For this review, take the finished solid that the model builds, in its own axes (mm). A direction names the side the tool comes from. Give positions to 0.01 mm unless a question says otherwise; leave off trailing zeros. One line per item, written item: value. Start each with the question number.
from build123d import *

# Parameters (mm, degrees)
SKETCH1_R            = 1
BOSS_EXTRUDE1_DEPTH  = 27.5
SKETCH2_R            = 1.01
BOSS_EXTRUDE2_DEPTH  = 13
SKETCH3_W            = 3.5
SKETCH3_H            = 13
BOSS_EXTRUDE3_DEPTH  = 49.6
SKETCH7_W            = 3.5
SKETCH7_H            = 49.5
BOSS_EXTRUDE6_DEPTH  = 5.5
SKETCH8_W            = 3.5
SKETCH8_H            = 49.5
BOSS_EXTRUDE7_DEPTH  = 14.5
FILLET2_R            = 4
BOSS_EXTRUDE8_DEPTH  = 29
BOSS_EXTRUDE9_DEPTH  = 0.2
BOSS_EXTRUDE11_DEPTH = 3.5
BOSS_EXTRUDE12_DEPTH = 1
FILLET2_OF_MIRROR1_R = 4
SKETCH15_R           = 1
CUT_EXTRUDE1_DEPTH   = 82.236014181
CHAMFER1_SIZE        = 0.5
FILLET3_R            = 0.5
FILLET4_R            = 0.5
FILLET6_R            = 0.7


with BuildPart() as part:
    # Sketch1 → Boss-Extrude1 (new body)
    with BuildSketch(Plane.XY):
        Circle(SKETCH1_R)
    boss_extrude1 = extrude(amount=BOSS_EXTRUDE1_DEPTH)


with BuildPart() as body_2:
    # Sketch2 → Boss-Extrude2 (new body)
    with BuildSketch(Plane.XY.offset(27.5)):
        with BuildLine():
            Line((-2.136524473, -0.092095918), (-4.5, -2.4))
            Line((-4.5, -2.4), (-1, -2.4))
            ThreePointArc((-1, -2.4), (-0.559963282, -2.050091796), (0, -2))
            ThreePointArc((0, -2), (1.487450997, 1.336970281), (-1.988677777, 0.212510468))
            ThreePointArc((-1.988677777, 0.212510468), (-2.036032236, 0.047311543), (-2.136524473, -0.092095918))
        make_face()
        Circle(SKETCH2_R, mode=Mode.SUBTRACT)
    boss_extrude2 = extrude(amount=-BOSS_EXTRUDE2_DEPTH)

    # Sketch3 → Boss-Extrude3 (add)
    with BuildSketch(Plane.XZ.offset(2.4)):
        with Locations((-2.75, 21)):
            Rectangle(SKETCH3_W, SKETCH3_H)
    boss_extrude3 = extrude(amount=BOSS_EXTRUDE3_DEPTH)

    # Sketch7 → Boss-Extrude6 (add)
    with BuildSketch(Plane.XY.offset(27.5)):
        with Locations((-2.75, -27.25)):
            Rectangle(SKETCH7_W, SKETCH7_H)
    boss_extrude6 = extrude(amount=BOSS_EXTRUDE6_DEPTH)

    # Sketch8 → Boss-Extrude7 (add)
    with BuildSketch(Plane(origin=(0, 0, 14.5), x_dir=(-1, 0, 0), z_dir=(0, 0, -1))):
        with Locations((2.75, -27.25)):
            Rectangle(SKETCH8_W, SKETCH8_H)
    boss_extrude7 = extrude(amount=BOSS_EXTRUDE7_DEPTH)

    # Fillet2
    fillet2_edges = [body_2.edges().sort_by_distance(p)[0] for p in [
        (-2.75, -2.5, 33),
        (-2.75, -52, 33),
    ]]
    fillet(fillet2_edges, radius=FILLET2_R)

    # Sketch10 → Boss-Extrude8 (add)
    with BuildSketch(Plane(origin=(0, 0, 0), x_dir=(-1, 0, 0), z_dir=(0, 0, -1))):
        Polygon((3.8, -52), (1, -52), (1, -54), (4.8, -54), (4.8, -53), (3.8, -53), align=None)
    boss_extrude8 = extrude(amount=-BOSS_EXTRUDE8_DEPTH)

    # Sketch11 → Boss-Extrude9 (add)
    with BuildSketch(Plane(origin=(-1, 0, 0), x_dir=(0, 0, -1), z_dir=(1, 0, 0))):
        with BuildLine():
            Line((0, -36.209762403), (-20, -36.209762403))
            ThreePointArc((-20, -36.209762403), (-21.414213562, -35.623975965), (-22, -34.209762403))
            Line((-22, -34.209762403), (-22, -25.209762403))
            ThreePointArc((-22, -25.209762403), (-21.414213562, -23.795548841), (-20, -23.209762403))
            Line((-20, -23.209762403), (0, -23.209762403))
            Line((0, -23.209762403), (0, -23.709762403))
            Line((0, -23.709762403), (-0.5, -23.709762403))
            Line((-0.5, -23.709762403), (-20, -23.709762403))
            ThreePointArc((-20, -23.709762403), (-21.060660172, -24.149102231), (-21.5, -25.209762403))
            Line((-21.5, -25.209762403), (-21.5, -34.209762403))
            ThreePointArc((-21.5, -34.209762403), (-21.060660172, -35.270422575), (-20, -35.709762403))
            Line((-20, -35.709762403), (-0.5, -35.709762403))
            Line((-0.5, -35.709762403), (0, -35.709762403))
            Line((0, -35.709762403), (0, -36.209762403))
        make_face()
    boss_extrude9 = extrude(amount=BOSS_EXTRUDE9_DEPTH)

    # Sketch13 → Boss-Extrude11 (add)
    with BuildSketch(Plane(origin=(-1, 0, 0), x_dir=(0, 0, -1), z_dir=(1, 0, 0))):
        with BuildLine():
            Line((-26.75, -5.5), (-0.75, -5.5))
            Line((-0.75, -5.5), (0, -5.5))
            Line((0, -5.5), (0, -4.75))
            Line((0, -4.75), (-26.75, -4.75))
            ThreePointArc((-26.75, -4.75), (-29.578427125, -5.921572875), (-30.75, -8.75))
            Line((-30.75, -8.75), (-30.75, -45.75))
            ThreePointArc((-30.75, -45.75), (-29.578427125, -48.578427125), (-26.75, -49.75))
            Line((-26.75, -49.75), (0, -49.75))
            Line((0, -49.75), (0, -49))
            Line((0, -49), (-0.75, -49))
            Line((-0.75, -49), (-26.75, -49))
            ThreePointArc((-26.75, -49), (-29.048097039, -48.048097039), (-30, -45.75))
            Line((-30, -45.75), (-30, -8.75))
            ThreePointArc((-30, -8.75), (-29.048097039, -6.451902961), (-26.75, -5.5))
        make_face()
    boss_extrude11 = extrude(amount=BOSS_EXTRUDE11_DEPTH)

    # Sketch14 → Boss-Extrude12 (add)
    with BuildSketch(Plane(origin=(2.5, 0, 0), x_dir=(0, 0, -1), z_dir=(1, 0, 0))):
        with BuildLine():
            Line((0, -49), (-26.75, -49))
            ThreePointArc((-26.75, -49), (-29.048097039, -48.048097039), (-30, -45.75))
            Line((-30, -45.75), (-30, -8.75))
            ThreePointArc((-30, -8.75), (-29.048097039, -6.451902961), (-26.75, -5.5))
            Line((-26.75, -5.5), (0, -5.5))
            Line((0, -5.5), (0, -4))
            Line((0, -4), (-26.75, -4))
            ThreePointArc((-26.75, -4), (-30.108757211, -5.391242789), (-31.5, -8.75))
            Line((-31.5, -8.75), (-31.5, -45.75))
            ThreePointArc((-31.5, -45.75), (-30.108757211, -49.108757211), (-26.75, -50.5))
            Line((-26.75, -50.5), (0, -50.5))
            Line((0, -50.5), (0, -49))
        make_face()
    boss_extrude12 = extrude(amount=BOSS_EXTRUDE12_DEPTH)


with BuildPart() as part_1:
    add(part.part)

    add(body_2.part)  # Mirror1 merges body 2
    # Mirror1: Boss-Extrude1, Boss-Extrude2, Boss-Extrude3, Boss-Extrude6, Boss-Extrude7, Boss-Extrude8, Boss-Extrude9, Boss-Extrude11, Boss-Extrude12 across plane
    add(boss_extrude1.mirror(Plane(origin=(0, 0, 0), x_dir=(1, 0, 0), z_dir=(0, 0, -1))))
    add(boss_extrude2.mirror(Plane(origin=(0, 0, 0), x_dir=(1, 0, 0), z_dir=(0, 0, -1))))
    add(boss_extrude3.mirror(Plane(origin=(0, 0, 0), x_dir=(1, 0, 0), z_dir=(0, 0, -1))))
    add(boss_extrude6.mirror(Plane(origin=(0, 0, 0), x_dir=(1, 0, 0), z_dir=(0, 0, -1))))
    add(boss_extrude7.mirror(Plane(origin=(0, 0, 0), x_dir=(1, 0, 0), z_dir=(0, 0, -1))))
    add(boss_extrude8.mirror(Plane(origin=(0, 0, 0), x_dir=(1, 0, 0), z_dir=(0, 0, -1))))
    add(boss_extrude9.mirror(Plane(origin=(0, 0, 0), x_dir=(1, 0, 0), z_dir=(0, 0, -1))))
    add(boss_extrude11.mirror(Plane(origin=(0, 0, 0), x_dir=(1, 0, 0), z_dir=(0, 0, -1))))
    add(boss_extrude12.mirror(Plane(origin=(0, 0, 0), x_dir=(1, 0, 0), z_dir=(0, 0, -1))))

    # Fillet2 of Mirror1
    fillet2_of_mirror1_edges = [part_1.edges().sort_by_distance(p)[0] for p in [
        (-2.75, -2.5, -33),
        (-2.75, -52, -33),
    ]]
    fillet(fillet2_of_mirror1_edges, radius=FILLET2_OF_MIRROR1_R)

    # Sketch15 → Cut-Extrude1 (cut, through all)
    with BuildSketch(Plane(origin=(0, 0, -27.5), x_dir=(-1, 0, 0), z_dir=(0, 0, -1))):
        Circle(SKETCH15_R)
    extrude(amount=-CUT_EXTRUDE1_DEPTH, mode=Mode.SUBTRACT)

    # Chamfer1
    chamfer1_edges = [part_1.edges().sort_by_distance(p)[0] for p in [
        (3.5, -4, 0),
        (3.5, -5.391242789, 30.108757211),
        (3.5, -27.25, 31.5),
        (3.5, -49.108757211, 30.108757211),
        (3.5, -50.5, 0),
        (3.5, -5.391242789, -30.108757211),
        (3.5, -27.25, -31.5),
        (3.5, -49.108757211, -30.108757211),
    ]]
    chamfer(chamfer1_edges, length=CHAMFER1_SIZE)

    # Fillet3
    fillet3_edges = [part_1.edges().sort_by_distance(p)[0] for p in [
        (2.5, -4, 0),
        (2.5, -5.391242789, 30.108757211),
        (2.5, -27.25, 31.5),
        (2.5, -49.108757211, 30.108757211),
        (2.5, -50.5, 0),
        (2.5, -49.108757211, -30.108757211),
        (2.5, -27.25, -31.5),
        (2.5, -5.391242789, -30.108757211),
    ]]
    fillet(fillet3_edges, radius=FILLET3_R - 0.0001)  # a hair under: the kernel refuses the full size

    # Fillet4
    fillet4_edges = [part_1.edges().sort_by_distance(p)[0] for p in [
        (-1, -49, 0),
        (-1, -48.048097039, 29.048097039),
        (-1, -27.25, 30),
        (-1, -6.451902961, 29.048097039),
        (-1, -5.5, 0),
        (-1, -48.048097039, -29.048097039),
        (-1, -27.25, -30),
        (-1, -6.451902961, -29.048097039),
    ]]
    fillet(fillet4_edges, radius=FILLET4_R)

    # Fillet6
    fillet6_edges = [part_1.edges().sort_by_distance(p)[0] for p in [
        (-4.5, -50.828427125, -31.828427125),
        (-4.5, -27.25, -33),
        (-4.5, -3.671572875, -31.828427125),
        (-4.5, -2.5, -28.25),
        (-4.5, -2.45, -27.5),
        (-4.5, -2.4, -21),
        (-4.5, -2.45, -14.5),
        (-4.5, -2.5, 0),
        (-4.5, -2.45, 14.5),
        (-4.5, -2.4, 21),
        (-4.5, -2.45, 27.5),
        (-4.5, -2.5, 28.25),
        (-4.5, -3.671572875, 31.828427125),
        (-4.5, -27.25, 33),
        (-4.5, -50.828427125, 31.828427125),
        (-4.5, -52, 0),
    ]]
    fillet(fillet6_edges, radius=FILLET6_R - 0.0001)  # a hair under: the kernel refuses the full size


solid = part_1.part
Q1. For faces 1 (the flat face through (-3, -53, -29)), 2 (the cylindrical face through (0.726, -48.547, 29.609)), 3 (the flat face through (-3, -53, 29)), list the 3-axis set-ups (+Z, -Z, +X, -X, +Y, -Y) from which the entire face can be reached by the end or side of a thin tool; tool diameter is ignored.
Q2. Mouldability with a two-part tool opening along Z and no side actions: class faces 4 (the conical face through (3.365, -5.615, 29.817)), 5 (the conical face through (3.365, -5.683, -29.885)), 6 (the flat face through (-1, -22, 0)) as pulls with the +Z half, pulls with the -Z half, needs draft (parallel to the pull), parting line crosses it, or undercut.
Q3. For line 1 along Y through (x, z) = (2.25, 2.5); line 2 along Z through (x, y) = (1.75, -28); line 3 along Y through (x, z) = (-2.75, -5.5), list the stretches that pass through material, from the lowest coordinate up.
Q4. For pin 1 Ø2 at (x, z) = (0.5, 15) entering from -Y; pin 2 Ø4.5 at (x, z) = (0.5, -6) entering from +Y; pin 3 Ø14.5 at (y, z) = (-28.5, -8.5) entering from +X, all flat-tipped, find the tip position at first contact; note any pin that passes through.
Answers below:
1. face 1: -Z, +X, -X, -Y
1. face 2: +Z, -Y
1. face 3: +Z, +X, -X, -Y
2. face 4: pulls with the +Z half
2. face 5: pulls with the -Z half
2. face 6: undercut
3. line 1: y = -49.75 to -49, -5.5 to -4.75
3. line 2: z = -30.75 to -30, 30 to 30.75
3. line 3: y = -54 to -2.5
4. pin 1: stops at y = -49.75
4. pin 2: stops at y = -2.5
4. pin 3: stops at x = -0.8
